from build123d import *

# Parameters (mm, degrees)
BOSS_EXTRUDE1_DEPTH          = 125
SKETCH2_R                    = 2
CUT_EXTRUDE1_DEPTH           = 144.165114466
FILLET1_R                    = 80
SKETCH3_R                    = 2.5
CUT_EXTRUDE2_DEPTH           = 10
CUT_EXTRUDE3_DEPTH           = 10
BASE_FLANGE1_START           = -3
BASE_FLANGE1_DEPTH           = 3
EDGE_FLANGE1_STRIP_W         = 19.4
EDGE_FLANGE1_STRIP_H         = 3
EDGE_FLANGE1_STRIP_CUT_DEPTH = 250
EDGE_FLANGE1_DEPTH           = 250
SKETCH13_R                   = 2
CUT_EXTRUDE4_DEPTH           = 10
SKETCH14_R                   = 2.5
CUT_EXTRUDE5_DEPTH           = 10


# Read off the part's stored shape, not the designer's step: Base-Flange1
# Sheet-metal steps are written as plain solids
with BuildPart() as part:
    # Sketch1 → Boss-Extrude1 (new, symmetric)
    with BuildSketch(Plane(origin=(0, 0, 0), x_dir=(0, 0, -1), z_dir=(1, 0, 0))):
        with BuildLine():
            Line((-31, 61.5), (-6, 61.5))
            ThreePointArc((-6, 61.5), (-0.343145751, 59.156854249), (2, 53.5))
            Line((2, 53.5), (2, -53.5))
            Line((2, -53.5), (-2, -53.5))
            Line((-2, -53.5), (-2, 53.5))
            ThreePointArc((-2, 53.5), (-3.171572875, 56.328427125), (-6, 57.5))
            Line((-6, 57.5), (-31, 57.5))
            Line((-31, 57.5), (-31, 61.5))
        make_face()
    extrude(amount=BOSS_EXTRUDE1_DEPTH, both=True)

    # Sketch2 → Cut-Extrude1 (cut, through all)
    with BuildSketch(Plane(origin=(0, 0, -2), x_dir=(-1, 0, 0), z_dir=(0, 0, -1))):
        with Locations(Location((60, 47, 0), (0, 0, 90))):
            Circle(SKETCH2_R)
        with Locations(Location((97.672105065, 25.25, 0), (0, 0, 90))):
            Circle(SKETCH2_R)
        with Locations(Location((97.672105065, -18.25, 0), (0, 0, 90))):
            Circle(SKETCH2_R)
        with Locations(Location((60, -40, 0), (0, 0, 90))):
            Circle(SKETCH2_R)
        with Locations(Location((22.327894935, -18.25, 0), (0, 0, 90))):
            Circle(SKETCH2_R)
        with Locations(Location((22.327894935, 25.25, 0), (0, 0, 90))):
            Circle(SKETCH2_R)
        with Locations(Location((-22.327894935, 25.25, 0), (0, 0, 90))):
            Circle(SKETCH2_R)
        with Locations(Location((-22.327894935, -18.25, 0), (0, 0, 90))):
            Circle(SKETCH2_R)
        with Locations(Location((-60, -40, 0), (0, 0, 90))):
            Circle(SKETCH2_R)
        with Locations(Location((-97.672105065, -18.25, 0), (0, 0, 90))):
            Circle(SKETCH2_R)
        with Locations(Location((-97.672105065, 25.25, 0), (0, 0, 90))):
            Circle(SKETCH2_R)
        with Locations(Location((-60, 47, 0), (0, 0, 90))):
            Circle(SKETCH2_R)
    extrude(amount=-CUT_EXTRUDE1_DEPTH, mode=Mode.SUBTRACT)

    # Fillet1
    fillet1_edges = [part.edges().sort_by_distance(p)[0] for p in [
        (125, -53.5, 0),
        (-125, -53.5, 0),
    ]]
    fillet(fillet1_edges, radius=FILLET1_R)

    # Sketch3 → Cut-Extrude2 (cut)
    with BuildSketch(Plane(origin=(0, 61.5, 0), x_dir=(1, 0, 0), z_dir=(0, 1, 0))):
        with Locations(Location((-112.5, -18.5, 0), (0, 0, 270))):
            Circle(SKETCH3_R)
        with Locations(Location((112.5, -18.5, 0), (0, 0, 270))):
            Circle(SKETCH3_R)
    extrude(amount=-CUT_EXTRUDE2_DEPTH, mode=Mode.SUBTRACT)

    # Sketch4 → Cut-Extrude3 (cut)
    with BuildSketch(Plane(origin=(0, 0, -2), x_dir=(-1, 0, 0), z_dir=(0, 0, -1))):
        with BuildLine():
            Line((6, 40.5), (6, 19.5))
            ThreePointArc((6, 19.5), (0, 13.5), (-6, 19.5))
            Line((-6, 19.5), (-6, 40.5))
            ThreePointArc((-6, 40.5), (0, 46.5), (6, 40.5))
        make_face()
    extrude(amount=-CUT_EXTRUDE3_DEPTH, mode=Mode.SUBTRACT)


with BuildPart() as body_2:
    # Base-Flange1 outline → Base-Flange1 (new body)
    with BuildSketch(Plane(origin=(0, 0, -2), x_dir=(-1, 0, 0), z_dir=(0, 0, -1)).offset(BASE_FLANGE1_START)):
        with BuildLine():
            Line((125, 65.5), (-125, 65.5))
            Line((-125, 65.5), (-125, 26.5))
            ThreePointArc((-125, 26.5), (-101.568542495, -30.068542495), (-45, -53.5))
            Line((-45, -53.5), (45, -53.5))
            ThreePointArc((45, -53.5), (101.568542495, -30.068542495), (125, 26.5))
            Line((125, 26.5), (125, 65.5))
        make_face()
    extrude(amount=BASE_FLANGE1_DEPTH)

    # Edge-Flange1 strip (across the edge) → Edge-Flange1 strip cut (cut)
    with BuildSketch(Plane(origin=(125, 65.5, 1), x_dir=(0, -1, 0), z_dir=(-1, 0, 0))):
        with Locations((-3, -1.5)):
            Rectangle(EDGE_FLANGE1_STRIP_W, EDGE_FLANGE1_STRIP_H)
    extrude(amount=EDGE_FLANGE1_STRIP_CUT_DEPTH, mode=Mode.SUBTRACT)

    # Edge-Flange1 section (across the edge) → Edge-Flange1 (add)
    with BuildSketch(Plane(origin=(125, 65.5, 1), x_dir=(0, -1, 0), z_dir=(-1, 0, 0))):
        with BuildLine():
            Line((0, 3.7), (0, 28.5))
            Line((0, 28.5), (3, 28.5))
            Line((3, 28.5), (3, 3.7))
            ThreePointArc((3, 3.7), (4.08370491, 1.08370491), (6.7, 0))
            Line((6.7, 0), (6.7, -3))
            ThreePointArc((6.7, -3), (1.962384566, -1.037615434), (0, 3.7))
        make_face()
    extrude(amount=EDGE_FLANGE1_DEPTH)

    # Sketch13 → Cut-Extrude4 (cut)
    with BuildSketch(Plane(origin=(0, 0, -2), x_dir=(-1, 0, 0), z_dir=(0, 0, -1))):
        with Locations(Location((97.672105065, -18.25, 0), (0, 0, 90))):
            Circle(SKETCH13_R)
        with Locations(Location((97.672105065, 25.25, 0), (0, 0, 90))):
            Circle(SKETCH13_R)
        with Locations(Location((60, 47, 0), (0, 0, 90))):
            Circle(SKETCH13_R)
        with Locations(Location((-97.672105065, -18.25, 0), (0, 0, 90))):
            Circle(SKETCH13_R)
        with Locations(Location((-60, -40, 0), (0, 0, 90))):
            Circle(SKETCH13_R)
        with Locations(Location((-22.327894935, -18.25, 0), (0, 0, 90))):
            Circle(SKETCH13_R)
        with Locations(Location((-22.327894935, 25.25, 0), (0, 0, 90))):
            Circle(SKETCH13_R)
        with Locations(Location((22.327894935, 25.25, 0), (0, 0, 90))):
            Circle(SKETCH13_R)
        with Locations(Location((22.327894935, -18.25, 0), (0, 0, 90))):
            Circle(SKETCH13_R)
        with Locations(Location((60, -40, 0), (0, 0, 90))):
            Circle(SKETCH13_R)
        with Locations(Location((-60, 47, 0), (0, 0, 90))):
            Circle(SKETCH13_R)
        with Locations(Location((-97.672105065, 25.25, 0), (0, 0, 90))):
            Circle(SKETCH13_R)
        with BuildLine():
            Line((6, 19.5), (6, 40.5))
            ThreePointArc((6, 40.5), (0, 46.5), (-6, 40.5))
            Line((-6, 40.5), (-6, 19.5))
            ThreePointArc((-6, 19.5), (0, 13.5), (6, 19.5))
        make_face()
    extrude(amount=-CUT_EXTRUDE4_DEPTH, mode=Mode.SUBTRACT)

    # Sketch14 → Cut-Extrude5 (cut)
    with BuildSketch(Plane(origin=(0, 65.5, 0), x_dir=(1, 0, 0), z_dir=(0, 1, 0))):
        with Locations(Location((-112.5, -17.5, 0), (0, 0, 270))):
            Circle(SKETCH14_R)
        with Locations(Location((112.5, -17.5, 0), (0, 0, 270))):
            Circle(SKETCH14_R)
    extrude(amount=-CUT_EXTRUDE5_DEPTH, mode=Mode.SUBTRACT)


solid = body_2.part
Verification items for the finished model (mm, model axes). A direction names the side the tool comes from. Round coordinates to 2 decimals unless told otherwise and drop trailing zeros. Loops run counter-clockwise (first coordinate to the right, second up) from the corner with the lowest first, then second, coordinate; pieces in that order, holes last. Notation, with made-up numbers: (-14.5, 1) - (31.5, 1) arc R30 ccw to (31.5, 40) - close; hole circle Ø6 at (3.25, -26). An arc over 180 degrees is marked (long way). Answer in a Markdown table with one row per item. Add a question column.
Q1. Section check B-B on x = -92. Enter the section's corners in (y, z), plus the area to 3 significant figures.
Q2. Material ranges on line 1 (X direction, y = 64, z = 17); line 2 (X direction, y = 25.25, z = -0.3); line 3 (Y direction, x = -55, z = 12.5), recorded low to high.
Q3. Release check for a two-part mould opening along Y. For faces 4 (the face through (1.75, 63.485, -0.089)), 5 (the face through (0.1, 13.5, -0.5)), 6 (the face through (2, 3, 1)) record: pulls with the +Y half, pulls with the -Y half, needs draft (parallel to the pull), parting line crosses it, or undercut.
Q4. Gauge pin test, flat ends, axial feed: pin 1 (2 mm diameter, centred on x = 16, z = 15, fed in from -Y); pin 2 (3 mm diameter, centred on x = -83, y = 41.5, fed in from +Z); pin 3 (5 mm diameter, centred on x = 41.5, z = 2.5, fed in from +Y). Record the tip position at first contact, or that the pin passes through.
Q5. Section check D-D on y = -2. Enter the section's corners in (x, z), plus the area to 3 significant figures.
Q6. Section check A-A on x = 112.5. Enter the section's corners in (y, z).
Q7. Section check C-C on z = 9.5. Enter the section's corners in (x, y), plus the area to 3 significant figures.
Q8. Tool access check on faces 1 (the face through (-0.1, 46.5, -0.5)), 2 (the face through (2, 62.5, 17)), 3 (the face through (2, 3, -2)). Record the directions out of +Z, -Z, +X, -X, +Y, -Y that give a thin tool (end or side, any length) a straight path to the whole face; none if there is none.
Found:
| question | item | result |
|---|---|---|
| 1 | outline | (-38.24, -2) - (58.8, -2) arc R6.7 ccw to (65.5, 4.7) - (65.5, 29.5) - (62.5, 29.5) - (62.5, 4.7) arc R3.7 cw to (58.8, 1) - (-38.24, 1) - close |
| 1 | area | 390 mm² |
| 2 | line 1 | x = -125 to -114.95, -110.05 to 110.05, 114.95 to 125 |
| 2 | line 2 | x = -124.99 to -99.67, -95.67 to -24.33, -20.33 to -6, 6 to 20.33, 24.33 to 95.67, 99.67 to 124.99 |
| 2 | line 3 | y = 62.5 to 65.5 |
| 3 | face 4 | pulls with the +Y half |
| 3 | face 5 | undercut |
| 3 | face 6 | needs draft |
| 4 | pin 1 | stops at y = 62.5 |
| 4 | pin 2 | stops at z = 1 |
| 4 | pin 3 | stops at y = 65.5 |
| 5 | outline | (-119.75, -2) - (119.75, -2) - (119.75, 1) - (-119.75, 1) - close |
| 5 | area | 719 mm² |
| 6 | outline | (-16.44, -2) - (58.8, -2) arc R6.7 ccw to (65.5, 4.7) - (65.5, 15) - (62.5, 15) - (62.5, 4.7) arc R3.7 cw to (58.8, 1) - (-16.44, 1) - close; (62.5, 20) - (65.5, 20) - (65.5, 29.5) - (62.5, 29.5) - close |
| 7 | outline | (-125, 62.5) - (125, 62.5) - (125, 65.5) - (-125, 65.5) - close |
| 7 | area | 750 mm² |
| 8 | face 1 | +Z, -Z |
| 8 | face 2 | +Z, +X, -X, -Y |
| 8 | face 3 | -Z, +X, -X, +Y, -Y |
